Could you check a few things on this model? Use its own coordinates, in mm. A direction names the side the tool comes from. Coordinates: 2 decimals unless noted, no trailing zeros. Write each loop counter-clockwise with the first axis right and the second up, starting at its lowest first coordinate (ties: lowest second). Pieces come first, ordered by that corner, then holes. Notation, with made-up numbers: (77, -6) - (104, -6) arc R12 cw to (104, 1) - close; hole circle Ø2 at (53, 42). An arc over 180 degrees is marked (long way). Answer as a JSON object with one key per item and string values. Group by question number.
1) Please list where these lines run through material, in increasing order: line 1 along X through (y, z) = (-2, 2.25); line 2 along Z through (x, y) = (1.25, 0); line 3 along Z through (x, y) = (13, -1).
2) We'd pull the mould along Y, two halves only. Please class faces 4 (the cylindrical face through (-1.775, -3.233, -1.341)), 5 (the flat face through (-3.014, -1.305, -0.74)), 6 (the flat face through (0, -2, -2)): released by +Y, released by -Y, zero draft, split by the parting line, or undercut.
3) On a 3-axis mill with a long thin cutter (end or side, diameter ignored), from which of +Z, -Z, +X, -X, +Y, -Y can I reach the whole of each face in a straight line? I mean faces 1 (the flat face through (-3, 0, -1.5)), 2 (the cylindrical face through (7, 0, -2)), 3 (the flat face through (15, 0, 0)). Say none if no direction works.
4) If we section it at A-A (x = 6.75): Write out the boundary of the cut face in (y, z), plus the area to 3 significant figures.
5) Will these pins go through, and if not, where does the flat tip stop? pin 1 Ø3 at (x, y) = (12.5, 1) entering from +Z; pin 2 Ø1 at (y, z) = (0.5, 0.5) entering from -X; pin 3 Ø3 at (x, y) = (2, 1) entering from -Z.
```python
from build123d import *

# Parameters (mm, degrees)
CHAMFER1_SIZE      = 0.4
CUT_EXTRUDE1_DEPTH = 2


with BuildPart() as part:
    # Sketch1 → Revolve1 (revolve)
    with BuildSketch(Plane.XY, mode=Mode.PRIVATE) as revolve1_sk:
        Polygon((-4, 0), (-4, 3.1), (-3.6, 3.5), (0, 3.5), (0, 2), (15, 2), (15, 0), align=None)
    revolve(revolve1_sk.sketch.rotate(Axis((15, 0, 0), (-1, 0, 0)), 180), axis=Axis((15, 0, 0), (-1, 0, 0)))

    # Chamfer1
    chamfer1_edges = [part.edges().sort_by_distance(p)[0] for p in [
        (15, 2, 0),
    ]]
    chamfer(chamfer1_edges, length=CHAMFER1_SIZE)

    # Sketch2 → Cut-Revolve1 (revolve, cut)
    with BuildSketch(Plane.XY, mode=Mode.PRIVATE) as cut_revolve1_sk:
        Polygon((-4, 0), (-4, 1.5), (-2, 1.5), (-1.598076211, 0), align=None)
    revolve(cut_revolve1_sk.sketch.rotate(Axis((-1.598076211, 0, 0), (-1, 0, 0)), 270), axis=Axis((-1.598076211, 0, 0), (-1, 0, 0)), mode=Mode.SUBTRACT)

    # Sketch3 → Cut-Extrude1 (cut)
    with BuildSketch(Plane(origin=(-4, 0, 0), x_dir=(0, 0, -1), z_dir=(1, 0, 0))):
        Polygon((-1.5, 0.866025404), (-1.5, -0.866025404), (0, -1.732050808), (1.5, -0.866025404), (1.5, 0.866025404), (0, 1.732050808), align=None)
    extrude(amount=CUT_EXTRUDE1_DEPTH, mode=Mode.SUBTRACT)


solid = part.part
```
Here are the results:
{
 "1": {"line 1": "x = -4 to 0", "line 2": "z = -2 to 2", "line 3": "z = -1.73 to 1.73"},
 "2": {"face 4": "split by the parting line", "face 5": "undercut", "face 6": "zero draft"},
 "3": {"face 1": "-X", "face 2": "+X", "face 3": "+Z, -Z, +X, +Y, -Y"},
 "4": {"outline": "circle Ø4 at (0, 0)", "area": "12.6 mm²"},
 "5": {"pin 1": "stops at z = 2", "pin 2": "stops at x = -1.92", "pin 3": "stops at z = -2"}
}
